The model under review builds one solid part; all positions refer to its coordinate system, in mm. Give positions to 0.01 mm unless a question says otherwise; leave off trailing zeros. Loops run counter-clockwise (first coordinate to the right, second up) from the corner with the lowest first, then second, coordinate; pieces in that order, holes last. Notation, with made-up numbers: (62.5, -3) -> (113.5, -3) arc R20 cw to (113.5, 21) -> close; hole circle Ø1 at (-6.5, 2.5). An arc over 180 degrees is marked (long way). Write each question's results on one line, items separated by ' | '. Start each with the question number.
Q1. We need section C-C (z = 15.5). Write out the cut boundary in (x, y), plus the area to 4 significant figures.
Q2. Insertion check: pin 1 Ø5 at (y, z) = (-21, -13.5) entering from +X; pin 2 Ø3 at (y, z) = (-10, -29) entering from -X; pin 3 Ø4 at (y, z) = (-18, -26) entering from +X; pin 4 Ø12 at (x, z) = (-36, -1.5) entering from +Y. Each pin has a flat end and moves straight along its axis. Give the tip position at first contact, or say it passes through.
Q3. We need section A-A (y = -16). Write out the cut boundary in (x, z).
Q4. Wall thickness on L1, parallel to X at y = -22.75, z = 25; L2, parallel to X at y = -14, z = -8: over which ranges is each line inside the solid? List them lowest first. Write a range as [from, to].
Q5. We need section B-B (x = 2.5). Write out the cut boundary in (y, z).
from build123d import *

# Parameters (mm, degrees)
F0_W     = 41.015632
F0_H     = 74.898109
F1_DEPTH = 25.4


with BuildPart() as f1:
    # F0 (on Front) → F1 (new body)
    with BuildSketch(Plane.XZ):
        with Locations((-25.85768, -5.349864)):
            Rectangle(F0_W, F0_H)
        Polygon((-58.402691, -42.798918), (-46.365496, -42.798918), (-46.365496, 32.099191), align=None)
        Polygon((-5.349864, 32.099191), (-5.349864, -42.798918), (6.687334, -42.798918), (15.157951, -42.798918), align=None)
    extrude(amount=F1_DEPTH)


solid = f1.part
Output:
1) outline: (-49.03, -25.4) -> (-0.8, -25.4) -> (-0.8, 0) -> (-49.03, 0) -> close | area: 1,225 mm2
2) pin 1: x = 7.82 | pin 2: x = -56.43 | pin 3: x = 11.11 | pin 4: y = 0
3) outline: (-58.4, -42.8) -> (15.16, -42.8) -> (-5.35, 32.1) -> (-46.37, 32.1) -> close
4) L1: [-47.51, -3.41] | L2: [-52.81, 5.63]
5) outline: (-25.4, -42.8) -> (0, -42.8) -> (0, 3.43) -> (-25.4, 3.43) -> close
